Read the model definition and answer for the solid it produces. Units are mm, in the model's axes. Face numbers are marked on the shaded views. A direction names the side the tool comes from. Coordinates: 2 decimals unless noted, no trailing zeros. Write each loop counter-clockwise with the first axis right and the second up, starting at its lowest first coordinate (ties: lowest second). Pieces come first, ordered by that corner, then holes. Notation, with made-up numbers: (9.25, 80) - (26.25, 80) arc R32 ccw to (26.25, 116) - close; hole circle Ø1 at (55, -14). An arc over 180 degrees is marked (long way). Return JSON: item names as keys, results as strings.
```python
from build123d import *

# Parameters (mm, degrees)
BOSS_EXTRUDE1_START = -10
BOSS_EXTRUDE1_DEPTH = 63
CHAMFER1_SIZE       = 0.5


# Read off the part's stored shape, not the designer's step: Boss-Extrude1
with BuildPart() as part:
    # Boss-Extrude1 outline → Boss-Extrude1 (new body)
    with BuildSketch(Plane(origin=(0, 0, 0), x_dir=(0, 0, -1), z_dir=(1, 0, 0)).offset(BOSS_EXTRUDE1_START)):
        Polygon((-4.04145, 6.999996736), (-8.0829, 0), (-4.04145, -6.999996736), (4.04145, -6.999996736), (8.0829, 0), (4.04145, 6.999996736), align=None)
    extrude(amount=BOSS_EXTRUDE1_DEPTH)

    # Sketch2 → Cut-Revolve1 (revolve, cut)
    with BuildSketch(Plane(origin=(0, 0, 0), x_dir=(1, 0, 0), z_dir=(0, 1, 0)), mode=Mode.PRIVATE) as cut_revolve1_sk:
        Polygon((0, 8.0829), (-10, 8.0829), (-10, 4), (-1, 4), (-1, 3.45), (0, 3.45), align=None)
    revolve(cut_revolve1_sk.sketch.rotate(Axis((-12.627683811, 0, 0), (1, 0, 0)), 180), axis=Axis((-12.627683811, 0, 0), (1, 0, 0)), mode=Mode.SUBTRACT)

    # Sketch3 → Cut-Revolve2 (revolve, cut)
    with BuildSketch(Plane(origin=(0, 0, 0), x_dir=(1, 0, 0), z_dir=(0, 1, 0)), mode=Mode.PRIVATE) as cut_revolve2_sk:
        Polygon((53, 8.0829), (53, 3), (45, 3), (45, 4), (19.9, 4), (19.9, 5), (18.9, 5), (18.9, 8.0829), align=None)
    revolve(cut_revolve2_sk.sketch.rotate(Axis((-14.24617289, 0, 0), (1, 0, 0)), 180), axis=Axis((-14.24617289, 0, 0), (1, 0, 0)), mode=Mode.SUBTRACT)

    # Chamfer1
    chamfer1_edges = [part.edges().sort_by_distance(p)[0] for p in [
        (-10, 0, -4),
        (53, 0, -3),
    ]]
    chamfer(chamfer1_edges, length=CHAMFER1_SIZE)


solid = part.part
```
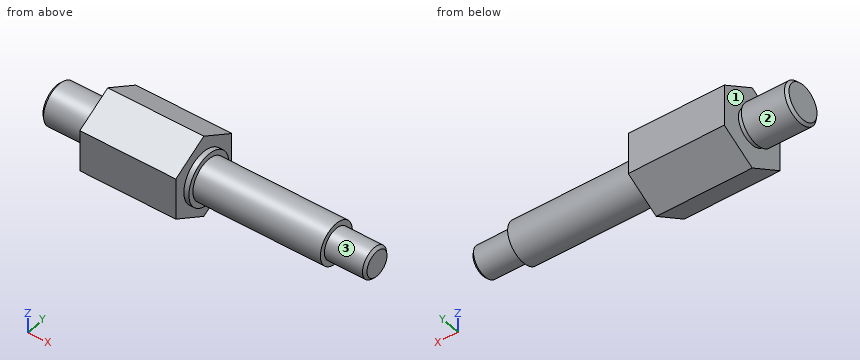
(1) A cutting plane is placed at A-A (z = 0). Determine the outline of the cut face in (x, y), and give its area (3 significant figures).
Answer:
{"outline": "(-10, -3.5) - (-9.5, -4) - (-1, -4) - (-1, -3.45) - (0, -3.45) - (0, -7) - (18.9, -7) - (18.9, -5) - (19.9, -5) - (19.9, -4) - (45, -4) - (45, -3) - (52.5, -3) - (53, -2.5) - (53, 2.5) - (52.5, 3) - (45, 3) - (45, 4) - (19.9, 4) - (19.9, 5) - (18.9, 5) - (18.9, 7) - (0, 7) - (0, 3.45) - (-1, 3.45) - (-1, 4) - (-9.5, 4) - (-10, 3.5) - close", "area": "602 mm²"}
(2) Which of the six approach directions +Z, -Z, +X, -X, +Y, -Y give full straight-line access (tool end or side, diameter ignored) to the marked faces 1, 2 and 3?
Answer:
{"face 1": "none", "face 2": "-X", "face 3": "+X"}
(3) A cutting plane is placed at C-C (y = -6). Determine the outline of the cut face in (x, z), and give its area (3 significant figures).
Answer:
{"outline": "(0, -4.62) - (18.9, -4.62) - (18.9, 4.62) - (0, 4.62) - close", "area": "175 mm²"}
(4) A cutting plane is placed at D-D (x = 29). Determine the outline of the cut face in (y, z), and give its area (3 significant figures).
Answer:
{"outline": "circle Ø8 at (0, 0)", "area": "50.3 mm²"}
(5) Flat-ended cylindrical pins translate along their axes: P1, Ø2, axis at x = 25.5, z = 1.5, coming from the +Y side; P2, Ø6, axis at x = 11.5, y = 4.5, coming from the -Z side; P3, Ø3, axis at x = 35.5, z = -2.5, coming from the +Y side. Find the tip coordinate at first contact, or state that the pin passes through.
Answer:
{"P1": "y = 3.97", "P2": "z = -7.22", "P3": "y = 3.87"}
(6) A cutting plane is placed at B-B (x = 7). Determine the outline of the cut face in (y, z), and give its area (3 significant figures).
Answer:
{"outline": "(-7, -4.04) - (0, -8.08) - (7, -4.04) - (7, 4.04) - (0, 8.08) - (-7, 4.04) - close", "area": "170 mm²"}
(7) Straight lines are drawn through the part: line 1 (X direction, y = -2.75, z = -1.75); line 2 (X direction, y = 2.25, z = -6); line 3 (Y direction, x = 1.5, z = 5.75). For each, find the intervals that lie inside material, in ascending order. Write a range as from..to.
Answer:
{"line 1": "-10..45", "line 2": "0..18.9", "line 3": "-4.04..4.04"}
